Autodesk Inventor part; units mm, degrees
ref_plane "YZ Plane" through (0, 0, 0) normal (1, 0, 0) x (0, 1, 0)
ref_plane "XZ Plane" through (0, 0, 0) normal (0, 1, 0) x (-1, 0, 0)
ref_plane "XY Plane" through (0, 0, 0) normal (0, 0, 1) x (1, 0, 0)
sketch "Sketch1" plane through (0, 0, 0) normal (0, 0, 1) x (1, 0, 0)
  circle A0 centre (0, 0) radius 25
  circle A1 centre (0, 0) radius 45
  dimension "d0" = 50
  dimension "d1" = 90
extrude "Extrusion1" add sketch "Sketch1" along normal mid plane 57
sketch "Sketch2" plane through (0, 0, 28.5) normal (0, 0, 1) x (1, 0, 0)
  circle A0 centre (0, 0) radius 100
  circle A1 centre (0, 0) radius 25
  dimension "d4" = 200
extrude "Extrusion2" add sketch "Sketch2" along normal blind 4
mirror "Mirror1" about plane through (0, 0, 0) normal (0, 0, 1) of "Extrusion2"
properties part number "filament spool"
Geometry: final body of the model. Coordinates: model frame, mm. A direction names the side the tool comes from. Coordinates: 2 decimals unless noted, no trailing zeros. Order: outer loops, then holes, each group sorted by start corner. A loop starts at its lowest first (then second) coordinate and runs counter-clockwise, first axis right, second up. Notation, with made-up numbers: (10.5, 37) - (57.5, 37) arc R23 cw to (57.5, 65) - close; hole circle Ø2 at (22, 26.25). An arc over 180 degrees is marked (long way). Use one line per item in the form item = value.
1) Pin query (flat end, axial travel): pin 1 (8 mm diameter, centred on y = -31, z = 16, fed in from -X); pin 2 (2 mm diameter, centred on y = 21, z = 4, fed in from -X); pin 3 (1.5 mm diameter, centred on y = -1, z = 20, fed in from -X). Return the tip coordinate at first contact, or that it passes through.
Solutions:
pin_1 = -36
pin_2 = -40.31
pin_3 = -45
2) Mould query, pull axis Z, two halves, no side actions, for faces 1 (the face through (21, -21, 32.5)), 2 (the face through (21, -43, 28.5)), 3 (the face through (-21, -21, -32.5)). Classes: +Z half, -Z half, draft (parallel to the pull), parting line (faces both ways), or undercut.
Solutions:
face_1 = +Z half
face_2 = undercut
face_3 = -Z half
3) Section C-C (z = 16). Return loops of the section in (x, y), then the cut area to 3 significant figures.
Solutions:
outline = circle Ø90 at (0, 0); hole circle Ø50 at (0, 0)
area = 4,400 mm^2
4) Section D-D (y = -66.5). Return loops of the section in (x, z).
Solutions:
outline = (-74.68, -32.5) - (74.68, -32.5) - (74.68, -28.5) - (-74.68, -28.5) - close; (-74.68, 28.5) - (74.68, 28.5) - (74.68, 32.5) - (-74.68, 32.5) - close
5) Set-up query: faces 4 (the face through (-21, -43, -28.5)), 5 (the face through (95.38, -30.04, 30.47)). Return all of +Z, -Z, +X, -X, +Y, -Y with unobstructed straight access to the full face (end or side cutting, diameter ignored); none if empty.
Solutions:
face_4 = none
face_5 = +Z, -Z
6) Ray query, L1, parallel to Y at x = 0, z = 1.5; L2, parallel to Z at x = 9, y = -84; L3, parallel to X at y = 3, z = -13.5. Return the intervals inside material, ascending.
Solutions:
L1 = -45 to -25, 25 to 45
L2 = -32.5 to -28.5, 28.5 to 32.5
L3 = -44.9 to -24.82, 24.82 to 44.9
7) Section A-A (y = 0). Return loops of the section in (x, z), then the cut area to 3 significant figures.
Solutions:
outline = (-100, -32.5) - (-25, -32.5) - (-25, 32.5) - (-100, 32.5) - (-100, 28.5) - (-45, 28.5) - (-45, -28.5) - (-100, -28.5) - close; (25, -32.5) - (100, -32.5) - (100, -28.5) - (45, -28.5) - (45, 28.5) - (100, 28.5) - (100, 32.5) - (25, 32.5) - close
area = 3,480 mm^2
